For this review, use the dimensioned drawing (mm, ordinates from the lowest corner) and the shaded views. Coordinates: 2 decimals unless noted, no trailing zeros. Order: outer loops, then holes, each group sorted by start corner. A loop starts at its lowest first (then second) coordinate and runs counter-clockwise, first axis right, second up. Notation, with made-up numbers: M 43.25,88.25 L 66.25,88.25 A24 cw 66.25,122.25 Z; hole C 5,43 d9. An arc over 180 degrees is marked long. Answer in a Markdown table with one row per item.
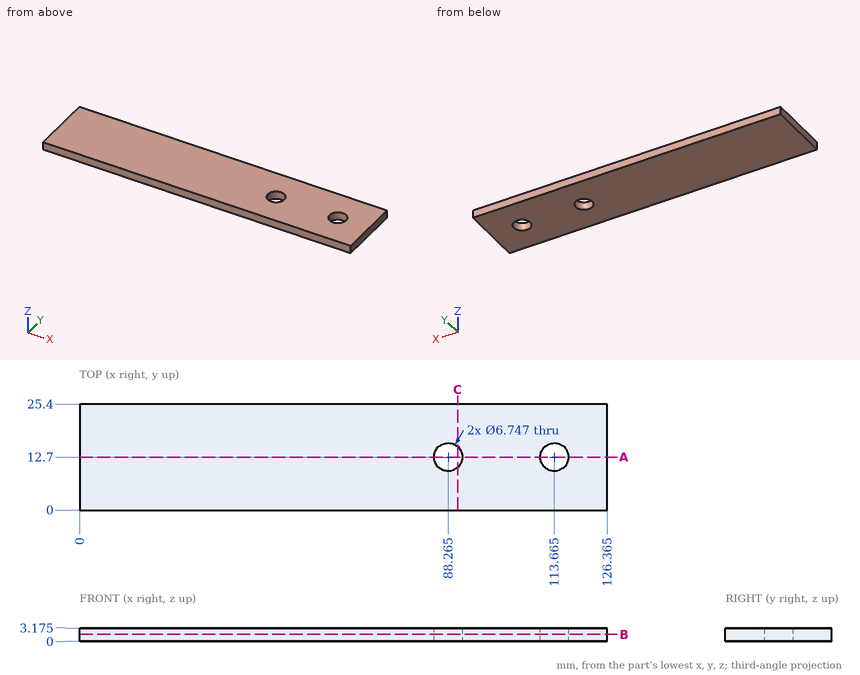
(1) Insertion check: P1, Ø5.5, axis at x = 88.265, y = 12.7, coming from the +Z side. The pin has a flat end and moves straight along its axis. Give the tip position at first contact, or say it passes through.
Report:
| item | result |
|---|---|
| P1 | through |
(2) Take a section at B-B (z = 1.7). Write out the cut boundary in (x, y) (1 decimal), then the cut area to 3 significant figures.
Report:
| item | result |
|---|---|
| outline | M 0,0 L 126.4,0 L 126.4,25.4 L 0,25.4 Z; hole C 88.3,12.7 d6.7; hole C 113.7,12.7 d6.7 |
| area | 3,140 mm^2 |
(3) Take a section at C-C (x = 90.5). Write out the cut boundary in (y, z) (1 decimal).
Report:
| item | result |
|---|---|
| outline | M 0,0 L 10.2,0 L 10.2,3.2 L 0,3.2 Z; M 15.2,0 L 25.4,0 L 25.4,3.2 L 15.2,3.2 Z |
(4) To check wall thickness, follow line 1 (X direction, y = 10, z = 1.45) (1 decimal); line 2 (Y direction, x = 90, z = 0.3); line 3 (X direction, y = 11, z = 2.25) (1 decimal). State the ranges of each line that lie inside material, in increasing order. Write a range as [from, to].
Report:
| item | result |
|---|---|
| line 1 | [0, 86.2], [90.3, 111.6], [115.7, 126.4] |
| line 2 | [0, 9.81], [15.59, 25.4] |
| line 3 | [0, 85.4], [91.2, 110.8], [116.6, 126.4] |
(5) Take a section at A-A (y = 12.7). Write out the cut boundary in (x, z) (1 decimal), then the cut area to 3 significant figures.
Report:
| item | result |
|---|---|
| outline | M 0,0 L 84.9,0 L 84.9,3.2 L 0,3.2 Z; M 91.6,0 L 110.3,0 L 110.3,3.2 L 91.6,3.2 Z; M 117,0 L 126.4,0 L 126.4,3.2 L 117,3.2 Z |
| area | 358 mm^2 |
